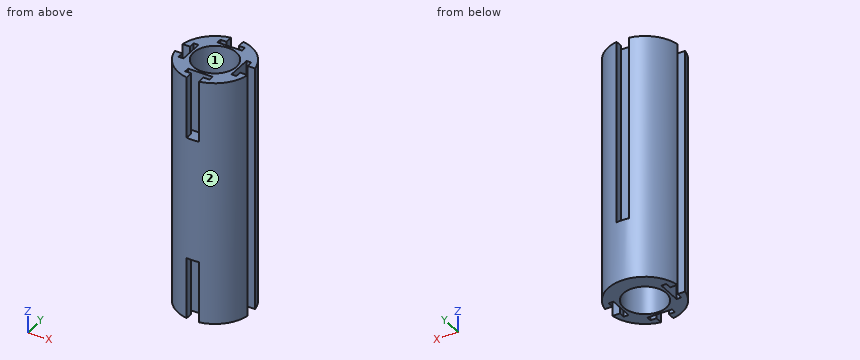
```python
from build123d import *

# Parameters (mm, degrees)
SKETCH1_R           = 30
SKETCH1_R_2         = 17.5
BOSS_EXTRUDE1_DEPTH = 200
CUT_EXTRUDE1_DEPTH  = 150
CUT_EXTRUDE2_DEPTH  = 50
CUT_EXTRUDE3_DEPTH  = 201


with BuildPart() as part:
    # Sketch1 → Boss-Extrude1 (new body)
    with BuildSketch(Plane.XY):
        Circle(SKETCH1_R)
        Circle(SKETCH1_R_2, mode=Mode.SUBTRACT)
    extrude(amount=BOSS_EXTRUDE1_DEPTH)

    # Sketch2 → Cut-Extrude1 (cut)
    with BuildSketch(Plane.XY.offset(200)):
        with BuildLine():
            Line((-10, 23.5), (-10, 19.5))
            Line((-10, 19.5), (10, 19.5))
            Line((10, 19.5), (10, 23.5))
            Line((10, 23.5), (5, 23.5))
            Line((5, 23.5), (5, 29.580398915))
            ThreePointArc((5, 29.580398915), (0, 30), (-5, 29.580398915))
            Line((-5, 29.580398915), (-5, 23.5))
            Line((-5, 23.5), (-10, 23.5))
        make_face()
    extrude(amount=-CUT_EXTRUDE1_DEPTH, mode=Mode.SUBTRACT)

    # Sketch2_3 → Cut-Extrude2 (cut)
    with BuildSketch(Plane.XY.offset(200)):
        with BuildLine():
            Line((-5, -23.5), (-5, -29.580398915))
            ThreePointArc((-5, -29.580398915), (0, -30), (5, -29.580398915))
            Line((5, -29.580398915), (5, -23.5))
            Line((5, -23.5), (10, -23.5))
            Line((10, -23.5), (10, -19.5))
            Line((10, -19.5), (-10, -19.5))
            Line((-10, -19.5), (-10, -23.5))
            Line((-10, -23.5), (-5, -23.5))
        make_face()
    cut_extrude2 = extrude(amount=-CUT_EXTRUDE2_DEPTH, mode=Mode.SUBTRACT)

    # Mirror1: Cut-Extrude2 across plane
    add(cut_extrude2.mirror(Plane.XY.offset(100)), mode=Mode.SUBTRACT)

    # Sketch2_5 → Cut-Extrude3 (cut, through all)
    with BuildSketch(Plane.XY.offset(200)):
        with BuildLine():
            Line((-23.5, 5), (-29.580398915, 5))
            ThreePointArc((-29.580398915, 5), (-30, 0), (-29.580398915, -5))
            Line((-29.580398915, -5), (-23.5, -5))
            Line((-23.5, -5), (-23.5, -10))
            Line((-23.5, -10), (-19.5, -10))
            Line((-19.5, -10), (-19.5, 10))
            Line((-19.5, 10), (-23.5, 10))
            Line((-23.5, 10), (-23.5, 5))
        make_face()
        with BuildLine():
            ThreePointArc((30, 0), (29.894915684, 2.508787808), (29.580398915, 5))
            Line((29.580398915, 5), (23.5, 5))
            Line((23.5, 5), (23.5, 10))
            Line((23.5, 10), (19.5, 10))
            Line((19.5, 10), (19.5, -10))
            Line((19.5, -10), (23.5, -10))
            Line((23.5, -10), (23.5, -5))
            Line((23.5, -5), (29.580398915, -5))
            ThreePointArc((29.580398915, -5), (29.894915684, -2.508787808), (30, 0))
        make_face()
    extrude(amount=-CUT_EXTRUDE3_DEPTH, mode=Mode.SUBTRACT)


solid = part.part
```
For this review, take the finished solid that the model builds, in its own axes (mm). Face numbers are marked on the shaded views. Round coordinates to 2 decimals unless told otherwise and drop trailing zeros. Write each loop counter-clockwise with the first axis right and the second up, starting at its lowest first coordinate (ties: lowest second). Pieces come first, ordered by that corner, then holes. Notation, with made-up numbers: (-30.5, 71) -> (16.5, 71) arc R18 cw to (16.5, 90) -> close; hole circle Ø7 at (-18, 70.25). An arc over 180 degrees is marked (long way). Use one line per item in the form item = value.
Q1. Consider section D-D (z = 110.5). State the section outline as (x, y) points.
Resolved:
outline = (-29.58, -5) arc R30 ccw to (29.58, -5) -> (23.5, -5) -> (23.5, -10) -> (19.5, -10) -> (19.5, 10) -> (23.5, 10) -> (23.5, 5) -> (29.58, 5) arc R30 ccw to (5, 29.58) -> (5, 23.5) -> (10, 23.5) -> (10, 19.5) -> (-10, 19.5) -> (-10, 23.5) -> (-5, 23.5) -> (-5, 29.58) arc R30 ccw to (-29.58, 5) -> (-23.5, 5) -> (-23.5, 10) -> (-19.5, 10) -> (-19.5, -10) -> (-23.5, -10) -> (-23.5, -5) -> close; hole circle Ø35 at (0, 0)
Q2. Clearance check with flat-ended pins moving along their axes: pin 1 Ø4.5 at (x, z) = (-22.5, 107.5) entering from +Y; pin 2 Ø3 at (x, z) = (-20.5, 142.5) entering from -Y; pin 3 Ø21 at (x, y) = (0, 0) entering from -Z; pin 4 Ø22 at (x, z) = (1.5, 157) entering from +Y. State where each tip first meets the part, or that it passes through.
Resolved:
pin_1 = 22.13
pin_2 = -23.22
pin_3 = through
pin_4 = 29.58
Q3. Consider section A-A (y = 0). State the section outline as (x, z) points, then the cut area to 3 significant figures.
Resolved:
outline = (-19.5, 0) -> (-17.5, 0) -> (-17.5, 200) -> (-19.5, 200) -> close; (17.5, 0) -> (19.5, 0) -> (19.5, 200) -> (17.5, 200) -> close
area = 800 mm²
Q4. The part is to be moulded in two halves that separate along X. For the marked faces 1 and 2, say which applies: released by +X, released by -X, zero draft, split by the parting line, or undercut.
Resolved:
face_1 = undercut
face_2 = split by the parting line
Q5. Consider section B-B (x = 0.5). State the section outline as (y, z) points.
Resolved:
outline = (-30, 50) -> (-19.5, 50) -> (-19.5, 0) -> (-17.49, 0) -> (-17.49, 200) -> (-19.5, 200) -> (-19.5, 150) -> (-30, 150) -> close; (17.49, 0) -> (30, 0) -> (30, 50) -> (19.5, 50) -> (19.5, 200) -> (17.49, 200) -> close
Q6. To check wall thickness, follow probe 1 along X at (y, z) = (5.5, 15.5); probe 2 along Y at (x, z) = (0, 46); probe 3 along X at (y, z) = (-22.5, 42). State the ranges of each line that lie inside material, in increasing order. Write a range as from..to.
Resolved:
probe_1 = -29.49..-23.5, -19.5..-16.61, 16.61..19.5, 23.5..29.49
probe_2 = -19.5..-17.5, 17.5..30
probe_3 = -19.84..-10, 10..19.84
